The model under review builds one solid part; all positions refer to its coordinate system, in mm. Face numbers are marked on the shaded views. A direction names the side the tool comes from. Round coordinates to 2 decimals unless told otherwise and drop trailing zeros. Loops run counter-clockwise (first coordinate to the right, second up) from the corner with the lowest first, then second, coordinate; pieces in that order, holes last. Notation, with made-up numbers: M 66.25,14.25 L 108.25,14.25 A22 cw 108.25,25.25 Z; hole C 65,45 d2. An arc over 180 degrees is marked long. Use a Markdown table: item, result. Add a question column.
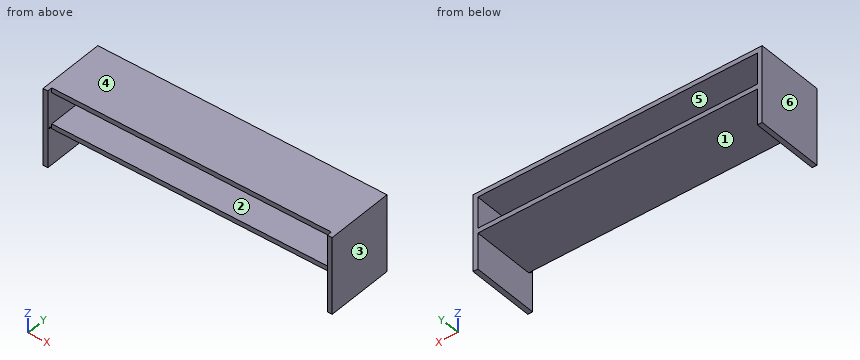
```python
from build123d import *

# Parameters (mm, degrees)
F0_W     = 1500
F0_H     = 350
F1_DEPTH = 25
F2_W     = 25
F2_H     = 350
F3_DEPTH = 375
F4_W     = 325
F4_H     = 25
F5_DEPTH = 1450
F6_R     = 4
F7_DEPTH = 735
F8_W     = 1450
F8_H     = 25
F9_DEPTH = 25


with BuildPart() as f1:
    # F0 (on Top) → F1 (new body)
    with BuildSketch(Plane.XY):
        Rectangle(F0_W, F0_H)
    extrude(amount=F1_DEPTH)

    # F2 (on face) → F3 (join)
    with BuildSketch(Plane(origin=(0, 0, 0), x_dir=(1, 0, 0), z_dir=(0, 0, -1))):
        with Locations((-737.5, 0)):
            Rectangle(F2_W, F2_H)
        with Locations((737.5, 0)):
            Rectangle(F2_W, F2_H)
    extrude(amount=F3_DEPTH)

    # F4 (on face) → F5 (join, through all)
    with BuildSketch(Plane.YZ.offset(-725)):
        with Locations((12.5, -175)):
            Rectangle(F4_W, F4_H)
    extrude(amount=F5_DEPTH)

    # F6 (on Right) → F7 (cut, symmetric)
    with BuildSketch(Plane.YZ):
        with Locations((-162.5, -175)):
            Circle(F6_R)
    extrude(amount=F7_DEPTH, both=True, mode=Mode.SUBTRACT)

    # F8 (on face) → F9 (cut)
    with BuildSketch(Plane.XY.offset(25)):
        with Locations((0, -162.5)):
            Rectangle(F8_W, F8_H)
    extrude(amount=-F9_DEPTH, mode=Mode.SUBTRACT)


solid = f1.part
```
(1) Consider section A-A, the plane z = -235. Give the boundary of the cut face in (x, y), then the cut area to 3 significant figures.
(2) To check wall thickness, follow probe 1 along X at (y, z) = (-40.5, -85); probe 2 along Z at (x, y) = (619, -94); probe 3 along Z at (x, y) = (-731.75, -162.5). State the ranges of each line that lie inside material, in increasing order.
(3) Insertion check: pin 1 Ø2 at (x, y) = (-595.5, 22) entering from -Z; pin 2 Ø7.5 at (x, z) = (212.5, 14.5) entering from -Y. Each pin has a flat end and moves straight along its axis. Give the tip position at first contact, or say it passes through.
(4) For the marked faces 1, 2 and 3, list the 3-axis set-ups (+Z, -Z, +X, -X, +Y, -Y) from which the entire face can be reached by the end or side of a thin tool; tool diameter is ignored.
(5) Consider section B-B, the plane y = 50. Give the boundary of the cut face in (x, z), then the cut area to 3 significant figures.
(6) Draft analysis for pull direction X (two halves, no side actions). For the marked faces 4, 5 and 6, state which applies: released by +X, released by -X, zero draft, split by the parting line, or undercut.
(7) Consider section C-C, the plane x = 80.5. Give the boundary of the cut face in (y, z), then the cut area to 4 significant figures.
Found:
| question | item | result |
|---|---|---|
| 1 | outline | M -750,-175 L -725,-175 L -725,175 L -750,175 Z; M 725,-175 L 750,-175 L 750,175 L 725,175 Z |
| 1 | area | 17,500 mm^2 |
| 2 | probe 1 | x = -750 to -725, 725 to 750 |
| 2 | probe 2 | z = -187.5 to -162.5, 0 to 25 |
| 2 | probe 3 | z = -375 to -179, -171 to 25 |
| 3 | pin 1 | stops at z = -187.5 |
| 3 | pin 2 | stops at y = -150 |
| 4 | face 1 | -Z, +Y, -Y |
| 4 | face 2 | +Y, -Y |
| 4 | face 3 | +Z, -Z, +X, +Y, -Y |
| 5 | outline | M -750,-375 L -725,-375 L -725,-187.5 L 725,-187.5 L 725,-375 L 750,-375 L 750,25 L -750,25 Z; hole M -725,-162.5 L 725,-162.5 L 725,0 L -725,0 Z |
| 5 | area | 92,500 mm^2 |
| 6 | face 4 | zero draft |
| 6 | face 5 | undercut |
| 6 | face 6 | released by -X |
| 7 | outline | M -150,-187.5 L 175,-187.5 L 175,-162.5 L -150,-162.5 Z; M -150,0 L 175,0 L 175,25 L -150,25 Z |
| 7 | area | 16,250 mm^2 |
